Check sheet for the modelled part. Datum: model origin and axes. Units: mm. A direction names the side the tool comes from. Coordinates: 2 decimals unless noted, no trailing zeros. Loops run counter-clockwise (first coordinate to the right, second up) from the corner with the lowest first, then second, coordinate; pieces in that order, holes last. Notation, with made-up numbers: M 59,36.25 L 64,36.25 A35 ccw 64,75.25 Z; hole C 28.25,41 d8. An arc over 180 degrees is marked long. Write each question's results on one line, items separated by ' | '. Start each with the question number.
from build123d import *

# Parameters (mm, degrees)
F0_W     = 80
F0_H     = 28
F0_W_2   = 60
F0_H_2   = 8
F0_W_3   = 56
F0_H_3   = 4
F1_DEPTH = 3
F2_DEPTH = 10
F3_R     = 5
F4_R     = 1


with BuildPart() as f1:
    # F0 (on Top) → F1 (new body)
    with BuildSketch(Plane.XY):
        Rectangle(F0_W, F0_H)
        Rectangle(F0_W_2, F0_H_2, mode=Mode.SUBTRACT)
        Rectangle(F0_W_2, F0_H_2)
        Rectangle(F0_W_3, F0_H_3, mode=Mode.SUBTRACT)
    extrude(amount=F1_DEPTH)

    # F0 (on Top) → F2 (join)
    with BuildSketch(Plane.XY):
        Rectangle(F0_W_2, F0_H_2)
        Rectangle(F0_W_3, F0_H_3, mode=Mode.SUBTRACT)
    extrude(amount=-F2_DEPTH)

    # F3
    f3_edges = [f1.edges().sort_by_distance(p)[0] for p in [
        (-40, 14, 1.5),
        (-40, -14, 1.5),
        (40, 14, 1.5),
        (40, -14, 1.5),
    ]]
    fillet(f3_edges, radius=F3_R)

    # F4
    f4_edges = [f1.edges().sort_by_distance(p)[0] for p in [
        (40, 0, 3),
        (38.535534, -12.535534, 3),
        (38.535534, 12.535534, 3),
        (0, -14, 3),
        (0, 14, 3),
        (-38.535534, -12.535534, 3),
        (-38.535534, 12.535534, 3),
        (-40, 0, 3),
        (0, 2, 3),
        (28, 0, 3),
        (0, -2, 3),
        (-28, 0, 3),
    ]]
    fillet(f4_edges, radius=F4_R)


solid = f1.part
Item 1: Thickness scan on line 1 (Y direction, x = -26.5, z = -6.5); line 2 (X direction, y = 1, z = -4); line 3 (Y direction, x = 24, z = 2). Record the ranges inside material, lowest first.
Item 2: Section check B-B (z = -3). Record the cut outline in (x, y).
Item 3: Section check A-A (x = 14.5). Record the cut outline in (y, z), plus the area to 3 significant figures.
Item 4: Release check for a two-part mould opening along X. For faces 1 (the face through (-38, -13, 1)), 2 (the face through (40, 0, 1)), 3 (the face through (0, -14, 1)), 4 (the face through (0, -2, -4)) record: +X half, -X half, draft (parallel to the pull), parting line (faces both ways), or undercut.
Item 5: Section check D-D (x = 33). Record the cut outline in (y, z), plus the area to 3 significant figures.
Item 6: Depth check by flat-ended pin: P1, Ø1.2, axis at y = -0.5, z = -5, coming from the -X side; P2, Ø3, axis at y = -2.5, z = -6, coming from the +X side; P3, Ø3, axis at x = 8, z = -3.5, coming from the +Y side. Enter the tip coordinate at first touch or a pass-through.
Item 7: Tool access check on faces 5 (the face through (0, 2, -4)), 6 (the face through (0, -4, -5)), 7 (the face through (0, 4, -5)), 8 (the face through (-30, 0, -5)). Record the directions out of +Z, -Z, +X, -X, +Y, -Y that give a thin tool (end or side, any length) a straight path to the whole face; none if there is none.
Item 8: Section check C-C (y = 7). Record the cut outline in (x, z).
Computed values:
1) line 1: y = -4 to -2, 2 to 4 | line 2: x = -30 to -28, 28 to 30 | line 3: y = -14 to -2, 2 to 14
2) outline: M -30,-4 L 30,-4 L 30,4 L -30,4 Z; hole M -28,-2 L 28,-2 L 28,2 L -28,2 Z
3) outline: M -14,0 L -4,0 L -4,-10 L -2,-10 L -2,2 A1 ccw -3,3 L -13,3 A1 ccw -14,2 Z; M 2,-10 L 4,-10 L 4,0 L 14,0 L 14,2 A1 ccw 13,3 L 3,3 A1 ccw 2,2 Z | area: 111 mm²
4) face 1: -X half | face 2: +X half | face 3: draft | face 4: undercut
5) outline: M -14,0 L 14,0 L 14,2 A1 ccw 13,3 L -13,3 A1 ccw -14,2 Z | area: 83.6 mm²
6) P1: stops at x = -30 | P2: stops at x = 30 | P3: stops at y = 4
7) face 5: +Z, -Z | face 6: -Z, +X, -X, -Y | face 7: -Z, +X, -X, +Y | face 8: -Z, -X, +Y, -Y
8) outline: M -40,0 L 40,0 L 40,2 A1 ccw 39,3 L -39,3 A1 ccw -40,2 Z
